Autodesk Inventor part; units mm, degrees
ref_plane "Work Plane1 top of part" through (0, 0, 9.525) normal (0, 0, 1) x (1, 0, 0)
sketch "Sketch1" plane through (0, 0, 0) normal (0, 0, 1) x (1, 0, 0)
  line L0 (-60.0075, 146.25) -> (60.0075, 146.25)
  line L1 (60.0075, 146.25) -> (60.0075, -12.5)
  line L2 (-60.0075, -12.5) -> (-60.0075, 146.25)
  line L3 (-60.0075, -12.5) -> (60.0075, -12.5)
  point P0 (0, 0)
  point P1 (0, -3.5617)
  point P2 (0, 146.25)
  dimension "d0" = 120.015
  dimension "d2" = 12.5
  dimension "d5" = 158.75
extrude "Extrusion1" add sketch "Sketch1" along normal blind 9.525
sketch "Sketch2" plane through (0, 0, 0) normal (0, 0, 1) x (1, 0, 0)
  circle A0 centre (-50, 0) radius 3.175
  circle A1 centre (50, 86.36) radius 3.175
  circle A2 centre (-50, 86.36) radius 3.175
  point P0 (0, 0)
  point P1 (50, 35.56)
  dimension "d6" = 6.35
  dimension "d8" = 50
  dimension "d28" = 86.36
  dimension "d29" = 50
  dimension "d128" = 50.8
hole "Hole1" at (-50, 0, 0) at (-50, 86.36, 0) at (50, 86.36, 0) direction (0, 0, 1) diameter 9.525 end through all
sketch "Sketch4" plane through (0, 0, 0) normal (0, 0, 1) x (1, 0, 0)
  line L0 (60.0075, -12.5) -> (-60.0075, -12.5)
  line L1 (0, 190.0524) -> (0, -46.2587)
  line L2 (-82.677, 0) -> (82.677, 0)
  line L3 (36.83, 110.944) -> (-36.83, 110.944)
  line L4 (-36.83, 110.944) -> (-36.83, -12.5)
  line L5 (36.83, 7.82) -> (60.0075, 7.82)
  line L6 (60.0075, 7.82) -> (60.0075, -12.5)
  line L7 (36.83, 7.82) -> (36.83, 110.944)
  line L8 (-36.83, -12.5) -> (60.0075, -12.5)
  line L9 (-60.0075, 146.25) -> (60.0075, 146.25)
  line L10 (0, -3.5649) -> (0, 156.2936)
  point P0 (0, 0)
  dimension "d30" = 123.444
  dimension "d31" = 20.32
  dimension "d32" = 35.306
  dimension "d112" = 73.66
  dimension "d132" = 36.83
  dimension "d133" = 36.83
extrude "Extrusion3" cut sketch "Sketch4" along normal up to next
sketch "Sketch5" plane through (0, 0, 0) normal (0, 0, 1) x (1, 0, 0)
  circle A0 centre (-50, 86.36) radius 4.7625
  circle A1 centre (50, 86.36) radius 4.7625
  circle A2 centre (-50, 0) radius 4.7625
  line L0 (-50, 86.36) -> (-50, 68.58) construction
  line L1 (-50, 0) -> (-50, 17.78) construction
  line L2 (50, 86.36) -> (50, 68.58) construction
  line L3 (-55.715, 74.295) -> (-44.285, 74.295)
  line L4 (-44.285, 74.295) -> (-44.285, 62.865)
  line L5 (-44.285, 62.865) -> (-55.715, 62.865)
  line L6 (-55.715, 62.865) -> (-55.715, 74.295)
  line L7 (-55.715, 23.495) -> (-44.285, 23.495)
  line L8 (-44.285, 23.495) -> (-44.285, 12.065)
  line L9 (-44.285, 12.065) -> (-55.715, 12.065)
  line L10 (-55.715, 12.065) -> (-55.715, 23.495)
  line L11 (44.285, 74.295) -> (55.715, 74.295)
  line L12 (55.715, 74.295) -> (55.715, 62.865)
  line L13 (55.715, 62.865) -> (44.285, 62.865)
  line L14 (44.285, 62.865) -> (44.285, 74.295)
  point P0 (0, 0)
  point P1 (-55.715, 68.58)
  point P2 (-50, 74.295)
  point P3 (-44.285, 17.78)
  point P4 (-50, 23.495)
  point P5 (55.715, 68.58)
  point P6 (50, 74.295)
  dimension "d36" = 17.78
  dimension "d38" = 11.43
  dimension "d39" = 11.43
  dimension "d63" = 50.8
  dimension "d97" = 17.78
  dimension "d98" = 17.78
extrude "Extrusion4" [suppressed]
fillet "Fillet2" [suppressed]
fillet "Fillet3" radius 12.7 2 edges at (36.83, 110.944, 4.7625) (-36.83, 110.944, 4.7625)
fillet "Fillet4" radius 3.175 6 edges at (36.83, 7.82, 4.7625) (60.0075, 146.25, 4.7625) (-60.0075, 146.25, 4.7625) (-60.0075, -12.5, 4.7625) (-36.83, -12.5, 4.7625) (60.0075, 7.82, 4.7625)
sketch "Sketch9" plane through (0, 0, 9.525) normal (0, 0, 1) x (1, 0, 0)
  circle A0 centre (-50, 86.36) radius 4.7625
  circle A1 centre (-50, 0) radius 4.7625
  circle A2 centre (50, 86.36) radius 4.7625
  line L0 (-50, 0) -> (-50, 140.9854) construction
  line L1 (50, 86.36) -> (50, 127.3454) construction
  circle A3 centre (-50, 43.18) radius 1.27 construction
  circle A4 centre (-50, 134.62) radius 1.27 construction
  circle A5 centre (51.6, 134.62) radius 1.5313 construction
  line L2 (-76.6675, 0) -> (76.6675, 0) construction
  point P0 (0, 0)
  dimension "d100" = 86.36
  dimension "d101" = 2.54
  dimension "d102" = 43.18
  dimension "d104" = 101.6
  dimension "d113" = 0
  dimension "d180" = 134.62
chamfer "Chamfer3" [suppressed]
chamfer "Chamfer4" distance 0.381 angle 45 6 edges at (-50, -4.7625, 9.525) (-50, 81.5975, 9.525) (50, 81.5975, 9.525) (-50, -4.7625, 0) (-50, 81.5975, 0) (50, 81.5975, 0)
sketch "Sketch10" plane through (0, 0, 0) normal (0, 0, 1) x (1, 0, 0)
  circle A0 centre (50, 86.36) radius 5.1435 construction
  line L0 (51.6, 134.62) -> (51.6, 24.6) construction
  line L1 (-76.6675, 0) -> (76.6675, 0) construction
  point P0 (0, 0)
  point P1 (-50, 134.62)
  point P2 (-50, 43.18)
  point P3 (-50, 43.18)
  point P4 (-50, 134.62)
  point P5 (-50, 134.62)
  dimension "d127" = 101.6
  dimension "d130" = 24.6
  dimension "d131" = 110.02
hole "Hole8 stdf holes flipped" at (51.6, 134.62, 0) at (-50, 134.62, 0) at (-50, 43.18, 0) at (51.6, 24.6, 0) direction (0, 0, 1) diameter 7.0358 end through all counterbore diameter 10.795 counterbore depth 6.35
sketch "Sketch11" plane through (0, 0, 0) normal (0, 0, 1) x (1, 0, 0)
  circle A0 centre (-50, 0) radius 4.7625
  circle A1 centre (-50, 86.36) radius 4.7625
  circle A2 centre (50, 86.36) radius 4.7625
  point P0 (0, 0)
  point P1 (-50, 25.019)
  point P2 (-50, 61.341)
  point P3 (50, 61.341)
  dimension "d134" = 25.019
  dimension "d135" = 25.019
  dimension "d136" = 25.019
hole "Hole9" at (50, 61.341, 0) at (-50, 61.341, 0) at (-50, 25.019, 0) direction (0, 0, 1) diameter 11.1125 end through all
sketch "Sketch13" plane through (0, 0, 0) normal (0, 0, -1) x (-1, 0, 0)
  circle A0 centre (50, 25.019) radius 5.5562
  line L0 (60.0075, -9.325) -> (60.0075, 143.075)
  line L1 (39.205, 35.814) -> (60.0075, 35.814)
  line L2 (60.0075, 35.814) -> (60.0075, 14.224)
  line L3 (60.0075, 14.224) -> (39.205, 14.224)
  line L4 (39.205, 14.224) -> (39.205, 35.814)
  circle A1 centre (50, 61.341) radius 5.5562
  line L5 (39.205, 72.136) -> (60.0075, 72.136)
  line L6 (60.0075, 72.136) -> (60.0075, 50.546)
  line L7 (60.0075, 50.546) -> (39.205, 50.546)
  line L8 (39.205, 50.546) -> (39.205, 72.136)
  point P0 (0, 0)
  dimension "d156" = 10.795
  dimension "d157" = 21.59
  dimension "d158" = 10.795
  dimension "d159" = 0
  dimension "d162" = 10.795
  dimension "d163" = 0
  dimension "d164" = 10.795
  dimension "d165" = 21.59
extrude "Extrusion5" cut sketch "Sketch13" against normal blind 2.54
sketch "Sketch14" plane through (0, 0, 2.54) normal (0, 0, -1) x (-1, 0, 0)
  circle A0 centre (50, 25.019) radius 5.5562
  circle A1 centre (50, 25.019) radius 9.5 construction
  circle A2 centre (50, 61.341) radius 5.5562 construction
  circle A3 centre (50, 61.341) radius 9.5 construction
  point P0 (0, 0)
  point P1 (43.283, 68.059)
  point P2 (56.717, 68.059)
  point P3 (56.717, 54.623)
  point P4 (43.283, 54.623)
  point P5 (43.283, 31.737)
  point P6 (56.717, 31.737)
  point P7 (56.717, 18.301)
  point P8 (43.283, 18.301)
  dimension "d166" = 19
  dimension "d167" = 19
  dimension "d168" = 13.4341
  dimension "d169" = 13.436
  dimension "d170" = 13.4341
  dimension "d171" = 13.436
hole "Hole11" at (-43.283, 18.301, 2.54) at (-43.283, 31.737, 2.54) at (-56.717, 31.737, 2.54) at (-56.717, 18.301, 2.54) at (-43.283, 54.623, 2.54) at (-43.283, 68.059, 2.54) at (-56.717, 68.059, 2.54) at (-56.717, 54.623, 2.54) direction (0, 0, 1) diameter 2.0066 depth 6.35 tip angle 118
fillet "Fillet5" radius 1.5875 8 edges at (-39.205, 14.224, 1.27) (-39.205, 35.814, 1.27) (-39.205, 50.546, 1.27) (-39.205, 72.136, 1.27) (-60.0075, 50.546, 1.27) (-60.0075, 72.136, 1.27) (-60.0075, 35.814, 1.27) (-60.0075, 14.224, 1.27)
sketch "Sketch15" plane through (0, 0, 0) normal (0, 0, -1) x (-1, 0, 0)
  line L0 (-60.0075, 143.075) -> (-60.0075, 10.995)
  circle A0 centre (-50, 61.341) radius 5.5562
  line L1 (-60.0075, 72.136) -> (-39.205, 72.136)
  line L2 (-39.205, 72.136) -> (-39.205, 50.546)
  line L3 (-39.205, 50.546) -> (-60.0075, 50.546)
  line L4 (-60.0075, 50.546) -> (-60.0075, 72.136)
  point P0 (0, 0)
  dimension "d181" = 21.59
  dimension "d182" = 10.795
  dimension "d183" = 10.795
extrude "Extrusion6" cut sketch "Sketch15" against normal blind 2.54
sketch "Sketch16" plane through (0, 0, 2.54) normal (0, 0, -1) x (-1, 0, 0)
  circle A0 centre (-50, 61.341) radius 5.5562
  line L0 (-56.7176, 68.0584) -> (-43.2831, 68.0584) construction
  line L1 (-43.2831, 68.0584) -> (-43.2831, 54.6239) construction
  line L2 (-43.2831, 54.6239) -> (-56.7176, 54.6239) construction
  line L3 (-56.7176, 54.6239) -> (-56.7176, 68.0584) construction
  circle A1 centre (-50, 61.341) radius 9.5 construction
  point P0 (0, 0)
  dimension "d198" = 19
  dimension "d199" = 13.4345
hole "Hole12" at (43.2831, 68.0584, 2.54) at (43.2831, 54.6239, 2.54) at (56.7176, 54.6239, 2.54) at (56.7176, 68.0584, 2.54) direction (0, 0, 1) diameter 2.0066 depth 6.35 tip angle 118
fillet "Fillet6" radius 1.5875 4 edges at (60.0075, 72.136, 1.27) (39.205, 50.546, 1.27) (60.0075, 50.546, 1.27) (39.205, 72.136, 1.27)
properties part number "J002887" material "ALUMINUM, 6061-T651"
Could you check a few things on this model? Use its own coordinates, in mm. A direction names the side the tool comes from. Coordinates: 2 decimals unless noted, no trailing zeros. Order: outer loops, then holes, each group sorted by start corner. A loop starts at its lowest first (then second) coordinate and runs counter-clockwise, first axis right, second up. Notation, with made-up numbers: M 80,-6 L 96,-6 A29 ccw 96,33 Z; hole C -15.5,69 d1. An arc over 180 degrees is marked long. Use a Markdown table: item, result. Add a question column.
Q1. We'd pull the mould along X, two halves only. Please class faces 1 (the flat face through (-60.008, 66, 5)), 2 (the flat face through (-49, -12.5, 5)), 3 (the cylindrical face through (51.363, 129.228, 3.219)): pulls with the +X half, pulls with the -X half, needs draft (parallel to the pull), parting line crosses it, or undercut.
Q2. I want a section at C-C on y = 0. List the corners of the cut face in (x, z) for me (1 decimal).
Q3. Which directions (+Z, -Z, +X, -X, +Y, -Y) give clear straight access to the entire face, cutting with the end or side of a thin tool? Please do faces 4 (the flat face through (-46, 43, 6.35)), 5 (the cylindrical face through (-51.431, 90.903, 4.824)), 6 (the cylindrical face through (-33.011, 107.322, 4.829)).
Q4. I'm going to push flat-ended pins straight in: pin 1 (10 mm diameter, centred on x = -38.5, y = 111.5, fed in from -Z); pin 2 (1.3 mm diameter, centred on x = 49.5, z = 1.5, fed in from -Y); pin 3 (1.8 mm diameter, centred on x = -43.283, y = 18.301, fed in from -Z); pin 4 (2.5 mm diameter, centred on x = 43.28, y = 54.62, fed in from -Z). Where does each tip first touch, or does it pass through?
Q5. If I drill on L1, parallel to X at y = 43.18, z = 3; L2, parallel to X at y = 134.62, z = 7; L3, parallel to X at y = 93.5, z = 7.5, over which ranges is the centre line in solid material (lowest first)?
Q6. I want a section at A-A on y = 43.18. Give the number of separate pieces and of enclosed holes in the cut face, then the cut area to 3 significant figures.
Q7. I want a section at B-B on y = 86.36. List the corners of the cut face in (x, z) for me (1 decimal).
Checked values:
| question | item | result |
|---|---|---|
| 1 | face 1 | pulls with the -X half |
| 1 | face 2 | needs draft |
| 1 | face 3 | undercut |
| 2 | outline | M -60,0 L -55.1,0 L -54.8,0.4 L -54.8,9.1 L -55.1,9.5 L -60,9.5 Z; M -45.2,0.4 L -44.9,0 L -36.8,0 L -36.8,9.5 L -44.9,9.5 L -45.2,9.1 Z |
| 3 | face 4 | -Z |
| 3 | face 5 | +Z, -Z |
| 3 | face 6 | +Z, -Z, -Y |
| 4 | pin 1 | z = 0 |
| 4 | pin 2 | y = 7.82 |
| 4 | pin 3 | z = 8.95 |
| 4 | pin 4 | z = 2.54 |
| 5 | L1 | -60.01 to -55.4, -44.6 to -36.83, 36.83 to 60.01 |
| 5 | L2 | -60.01 to -53.52, -46.48 to 48.08, 55.12 to 60.01 |
| 5 | L3 | -60.01 to -36.83, 36.83 to 60.01 |
| 6 | separate pieces | 3 |
| 6 | enclosed holes | 0 |
| 6 | area | 351 mm² |
| 7 | outline | M -60,0 L -55.1,0 L -54.8,0.4 L -54.8,9.1 L -55.1,9.5 L -60,9.5 Z; M -45.2,0.4 L -44.9,0 L -36.8,0 L -36.8,9.5 L -44.9,9.5 L -45.2,9.1 Z; M 36.8,0 L 44.9,0 L 45.2,0.4 L 45.2,9.1 L 44.9,9.5 L 36.8,9.5 Z; M 54.8,0.4 L 55.1,0 L 60,0 L 60,9.5 L 55.1,9.5 L 54.8,9.1 Z |
